Verification items for this drawing (mm, ordinates from the low corner). Give positions to 0.01 mm unless a question says otherwise; leave off trailing zeros. Write each loop counter-clockwise with the first axis right and the second up, starting at its lowest first coordinate (ties: lowest second). Pieces come first, ordered by that corner, then holes. Notation, with made-up numbers: (84.25, 34) -> (118.25, 34) arc R20 cw to (118.25, 57) -> close; hole circle Ø11 at (-32.75, 76.5). An arc over 180 degrees is marked (long way). One line per item, written item: value.
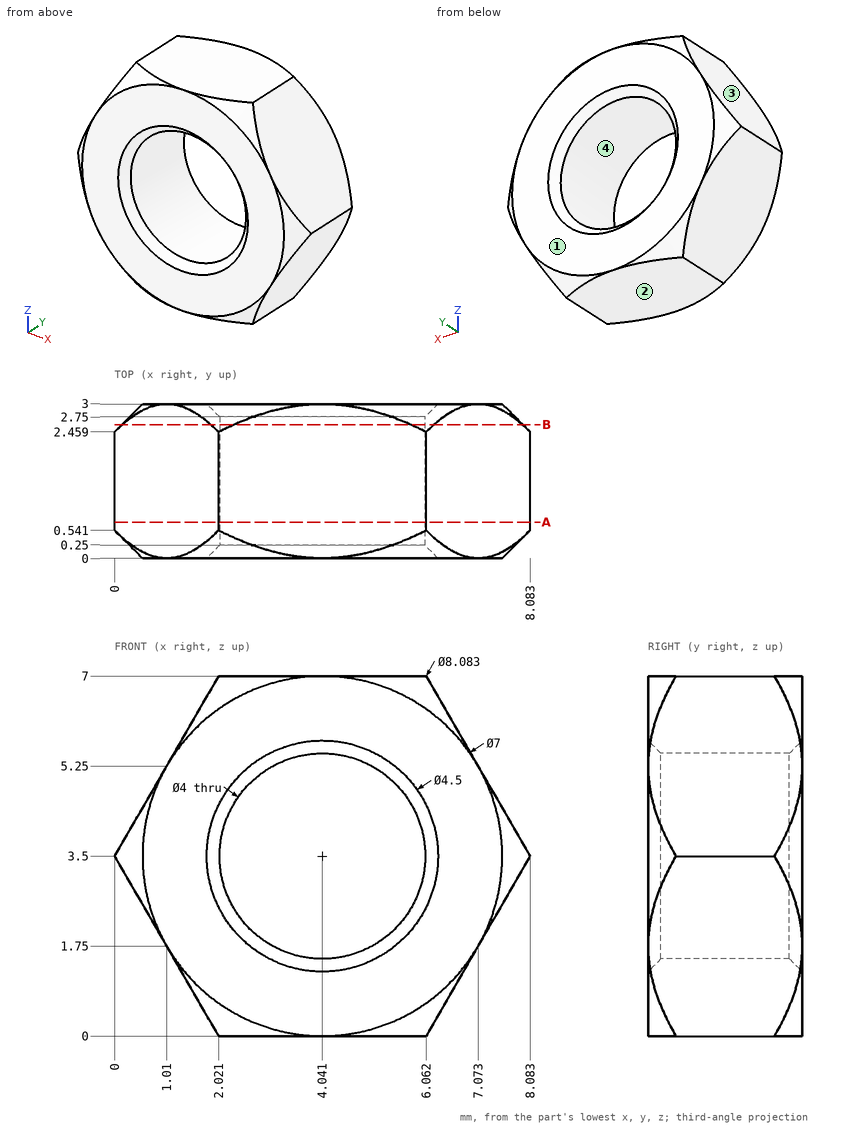
1) Depth check by flat-ended pin: pin 1 Ø3 at (x, z) = (4.5, 3) entering from +Y. Enter the tip coordinate at first touch or a pass-through.
Verdict:
pin 1: y = 2.93
2) Sectioned sample at B-B on y = 2.6. Record the cut outline in (x, z).
Verdict:
outline: (0.15, 3.24) -> (1.87, 0.26) arc R3.9 ccw to (2.32, 0) -> (5.76, 0) arc R3.9 ccw to (6.21, 0.26) -> (7.93, 3.24) arc R3.9 ccw to (7.93, 3.76) -> (6.21, 6.74) arc R3.9 ccw to (5.76, 7) -> (2.32, 7) arc R3.9 ccw to (1.87, 6.74) -> (0.15, 3.76) arc R3.9 ccw to start; hole circle Ø4 at (4.04, 3.5)
3) Mould release check, pull along Z, two halves, no side actions. Record for the marked faces 1, 2, 3 and 4: released by +Z, released by -Z, zero draft, split by the parting line, or undercut.
Verdict:
face 1: zero draft
face 2: released by -Z
face 3: released by +Z
face 4: undercut
4) Sectioned sample at A-A on y = 0.7. Record the cut outline in (x, z).
Verdict:
outline: (0, 3.5) -> (2.02, 0) -> (6.06, 0) -> (8.08, 3.5) -> (6.06, 7) -> (2.02, 7) -> close; hole circle Ø4 at (4.04, 3.5)
5) Scan lines: probe 1 along Z at (x, y) = (4, 1.15); probe 2 along X at (y, z) = (0.9, 2) (1 decimal); probe 3 along X at (y, z) = (0.5, 4.5) (1 decimal). Record each from-to range of solid material in increasing order.
Verdict:
probe 1: 0 to 1.5, 5.5 to 7
probe 2: 0.9 to 2.7, 5.4 to 7.2
probe 3: 0.6 to 2.3, 5.8 to 7.5
